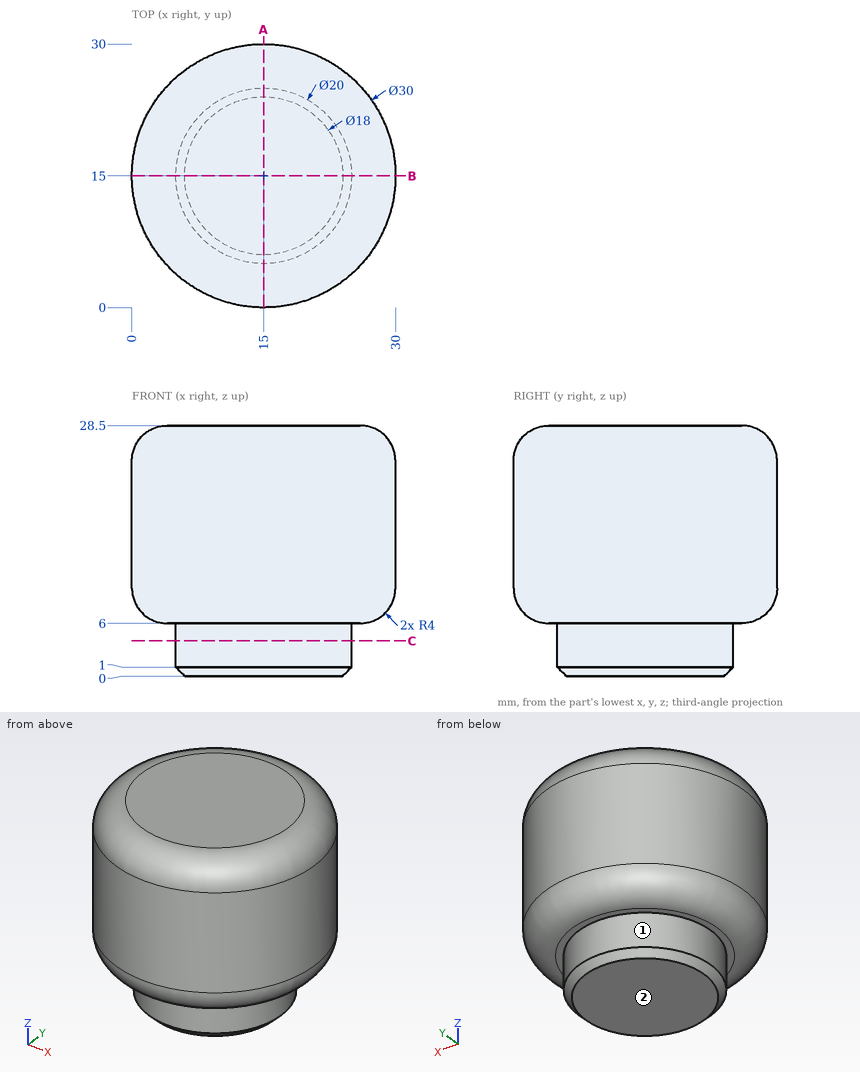
Design review of the part shown in the three views and the two pictorial views. Dimensions are in mm from the part's minimum x, y and z. A direction names the side the tool comes from. Coordinates: 2 decimals unless noted, no trailing zeros. Write each loop counter-clockwise with the first axis right and the second up, starting at its lowest first coordinate (ties: lowest second). Pieces come first, ordered by that corner, then holes.
1) We need section C-C on z = 4. State the section outline as (x, y) points, then the cut area to 3 significant figures.
2) We need section A-A on x = 15. State the section outline as (y, z) points, then the cut area to 3 significant figures.
3) Clearance check with flat-ended pins moving along their axes: pin 1 Ø8 at (x, z) = (8, 24) entering from -Y; pin 2 Ø1.5 at (x, z) = (17.5, 22) entering from -Y; pin 3 Ø1 at (y, z) = (15.5, 25) entering from +X. State where each tip first meets the part, or that it passes through.
4) To check wall thickness, follow probe 1 along Z at (x, y) = (5, 17.5); probe 2 along Y at (x, z) = (15, 4.5). State the ranges of each line that lie inside material, in increasing order.
5) Machinability: for the marked faces 1 and 2, which of the approach directions +Z, -Z, +X, -X, +Y, -Y give a long, thin tool a straight path to every point of the face, cutting with its end or side? Answer none if there is none.
Answer list:
1. outline: circle Ø20 at (15, 15)
1. area: 314 mm2
2. outline: (0, 10) arc R4 ccw to (4, 6) - (5, 6) - (5, 1) - (6, 0) - (24, 0) - (25, 1) - (25, 6) - (26, 6) arc R4 ccw to (30, 10) - (30, 24.5) arc R4 ccw to (26, 28.5) - (4, 28.5) arc R4 ccw to (0, 24.5) - close
2. area: 780 mm2
3. pin 1: stops at y = 0.3
3. pin 2: stops at y = 0.1
3. pin 3: stops at x = 30
4. probe 1: z = 6 to 28.5
4. probe 2: y = 5 to 25
5. face 1: -Z
5. face 2: -Z, +X, -X, +Y, -Y
